```python
from build123d import *

# Parameters (mm, degrees)
ELECTRONICS_GLASS_EXTRUDE_DEPTH = 2050


with BuildPart() as part:
    # Electronics Glass Sketch → Electronics Glass Extrude (new body)
    with BuildSketch(Plane(origin=(0, 0, 0), x_dir=(1, 0, 0), z_dir=(0, 1, 0))):
        with BuildLine():
            Line((616.097304934, -129.692986908), (505.548652467, -654.846493454))
            Line((505.548652467, -654.846493454), (485.977581789, -650.726639994))
            Line((485.977581789, -650.726639994), (596.526234256, -125.573133448))
            ThreePointArc((596.526234256, -125.573133448), (606.322749203, -63.125936022), (609.6, 0))
            ThreePointArc((609.6, 0), (0, 609.6), (-609.6, 0))
            ThreePointArc((-609.6, 0), (-606.322749203, -63.125936022), (-596.526234256, -125.573133448))
            Line((-596.526234256, -125.573133448), (-485.977581789, -650.726639994))
            Line((-485.977581789, -650.726639994), (-505.548652467, -654.846493454))
            Line((-505.548652467, -654.846493454), (-616.097304934, -129.692986908))
            ThreePointArc((-616.097304934, -129.692986908), (0, 629.6), (616.097304934, -129.692986908))
        make_face()
    extrude(amount=ELECTRONICS_GLASS_EXTRUDE_DEPTH)


solid = part.part
```
For this review, take the finished solid that the model builds, in its own axes (mm). A direction names the side the tool comes from. Give positions to 0.01 mm unless a question says otherwise; leave off trailing zeros. Order: outer loops, then holes, each group sorted by start corner. A loop starts at its lowest first (then second) coordinate and runs counter-clockwise, first axis right, second up.
1) Take a section at B-B (y = 325). Give the boundary of the cut face in (x, z), then the cut area to 3 significant figures.
2) Take a section at A-A (x = 549). Give the boundary of the cut face in (y, z), then the cut area to 3 significant figures.
3) Take a section at C-C (x = 0). Give the boundary of the cut face in (y, z), then the cut area to 3 significant figures.
4) For faces 1 (the face through (540.478, 1010.65, 391.826)), 2 (the face through (329, 0, -514)), list the 3-axis set-ups (+Z, -Z, +X, -X, +Y, -Y) from which the entire face can be reached by the end or side of a thin tool; tool diameter is ignored.
5) Take a section at D-D (x = -138). Give the boundary of the cut face in (y, z), then the cut area to 3 significant figures.
6) The part is to be moulded in two halves that separate along Z. For faces 3 (the face through (561.597, 1010.65, 388.594)), 4 (the face through (-542.026, 1010.65, 384.474)), 5 (the face through (329, 2050, -514)), say which applies: released by +Z, released by -Z, zero draft, split by the parting line, or undercut.
7) Wall thickness on line 1 (Z direction, x = -127.5, y = 1441.5); line 2 (X direction, y = 1026.5, z = -502.5); line 3 (X direction, y = 1311, z = 130.5): over which ranges is each line inside the solid? List them lowest first.
8) Insertion check: pin 1 (10 mm diameter, centred on y = 1629.5, z = 475, fed in from -X); pin 2 (6 mm diameter, centred on y = 1719, z = -92.5, fed in from +X); pin 3 (6 mm diameter, centred on y = 1115.5, z = 363, fed in from +X). Each pin has a flat end and moves straight along its axis. Give the tip position at first contact, or say it passes through.
Derived:
1. outline: (-616.1, 129.69) arc R629.6 ccw (long way) to (616.1, 129.69) - (505.55, 654.85) - (485.98, 650.73) - (596.53, 125.57) arc R609.6 cw (long way) to (-596.53, 125.57) - (-485.98, 650.73) - (-505.55, 654.85) - close
1. area: 65,500 mm2
2. outline: (0, -308.21) - (2050, -308.21) - (2050, -264.97) - (0, -264.97) - close; (0, 351.34) - (2050, 351.34) - (2050, 448.43) - (0, 448.43) - close
2. area: 288,000 mm2
3. outline: (0, -629.6) - (2050, -629.6) - (2050, -609.6) - (0, -609.6) - close
3. area: 41,000 mm2
4. face 1: +Y, -Y
4. face 2: +Z, -Z, +X, -X, -Y
5. outline: (0, -614.29) - (2050, -614.29) - (2050, -593.77) - (0, -593.77) - close
5. area: 42,100 mm2
6. face 3: released by +Z
6. face 4: undercut
6. face 5: zero draft
7. line 1: z = -616.55 to -596.12
7. line 2: x = -379.33 to -345.12, 345.12 to 379.33
7. line 3: x = -615.93 to -595.49, 595.49 to 615.93
8. pin 1: stops at x = -544.46
8. pin 2: stops at x = 623.21
8. pin 3: stops at x = 567.62
